```python
from build123d import *

# Parameters (mm, degrees)
F0_R     = 1.4
F1_DEPTH = 40
F2_W     = 3.4122867597
F2_H     = 22.5
F3_DEPTH = 25
F5_DEPTH = 2.75
F4_R     = 1.75
F4_R_2   = 19
F6_DEPTH = 25


with BuildPart() as f1:
    # F0 (on Top) → F1 (new body)
    with BuildSketch(Plane.XY):
        Polygon((-1.5877132403, -2.75), (1.5877132403, -2.75), (3.17543, 0), (1.5877132403, 2.75), (-3.3508529611, 5.5), (-46.7631397208, 5.5), (-46.7631397208, 2.75), (-4.7631397208, 2.75), (-3.1754264805, 0), align=None)
        Circle(F0_R, mode=Mode.SUBTRACT)
    extrude(amount=F1_DEPTH)

    # F2 (on face) → F3 (cut)
    with BuildSketch(Plane(origin=(0, 5.5, 0), x_dir=(-1, 0, 0), z_dir=(0, 1, 0))):
        Polygon((6.7631397208, 40.8263410057), (-4.1816732138, 40.8263410057), (-4.1816732138, 17.5), (3.3508529611, 17.5), (3.3508529611, 40), (6.7631397208, 40), align=None)
        with Locations((5.056996341, 28.75)):
            Rectangle(F2_W, F2_H)
    extrude(amount=-F3_DEPTH, mode=Mode.SUBTRACT)

    # F4 (on face) → F5 (join)
    with BuildSketch(Plane.XZ.offset(-2.75)):
        with BuildLine():
            Line((-46.7631397208, 9.692235936), (-46.7631397208, 30.307764064))
            ThreePointArc((-46.7631397208, 30.307764064), (-49.2631397208, 20), (-46.7631397208, 9.692235936))
        make_face()
        with BuildLine():
            ThreePointArc((-16.4553756568, 40), (-26.7631397208, 42.5), (-37.0709037849, 40))
            Line((-37.0709037849, 40), (-16.4553756568, 40))
        make_face()
    extrude(amount=-F5_DEPTH)

    # F4 (on face) → F6 (cut)
    with BuildSketch(Plane.XZ.offset(-2.75)):
        with BuildLine():
            Line((-6.7631397208, 40), (-9.7631397208, 40))
            ThreePointArc((-9.7631397208, 40), (-7.6418193773, 39.1213203436), (-6.7631397208, 37))
            Line((-6.7631397208, 37), (-6.7631397208, 40))
        make_face()
        with BuildLine():
            ThreePointArc((-46.7631397208, 37), (-45.8844600644, 39.1213203436), (-43.7631397208, 40))
            Line((-43.7631397208, 40), (-46.7631397208, 40))
            Line((-46.7631397208, 40), (-46.7631397208, 37))
        make_face()
        with Locations((-42.6730422975, 35.9099025767)):
            Circle(F4_R)
        with Locations((-42.6730422975, 4.0900974233)):
            Circle(F4_R)
        with Locations((-10.8532371441, 4.0900974233)):
            Circle(F4_R)
        with Locations((-10.8532371441, 35.9099025767)):
            Circle(F4_R)
        with Locations((-26.7631397208, 20)):
            Circle(F4_R_2)
    extrude(amount=-F6_DEPTH, mode=Mode.SUBTRACT)


solid = f1.part
```
Geometry: final body of the model. Coordinates: model frame, mm. A direction names the side the tool comes from. Round coordinates to 2 decimals unless told otherwise and drop trailing zeros. Order: outer loops, then holes, each group sorted by start corner. A loop starts at its lowest first (then second) coordinate and runs counter-clockwise, first axis right, second up. Notation, with made-up numbers: (77, 20) -> (135, 20) arc R17 ccw to (135, 26) -> close; hole circle Ø6 at (33.25, 88.5). An arc over 180 degrees is marked (long way). Use CSV: the item, a comma, the result in double quotes. Start each with the question number.
1) Section B-B (z = 13). Return the cut outline in (x, y), and give its area (3 significant figures).
2) Section C-C (x = 0). Return the cut outline in (y, z).
3) Draft query along Z for faces 4 (the face through (-9.184, 4.106, 36.436)), 5 (the face through (-0.847, 4.106, 8.628)), 6 (the face through (-46, 4, 39)), 7 (the face through (-44.42, 4.11, 4.17)). Return one class per face: +Z half, -Z half, draft (parallel to the pull), parting line (faces both ways), or undercut.
4) Section D-D (y = 4.75). Return the cut outline in (x, z), and give its area (3 significant figures).
5) Section A-A (z = 20). Return the cut outline in (x, y), and give its area (3 significant figures).
6) Material intervals for line 1 along X through (y, z) = (4, 4); line 2 along X through (y, z) = (-0.75, 9); line 3 along X through (y, z) = (4.75, 7), sorted ascending. Write a range as from..to.
7) First-contact query: pin 1 Ø2 at (x, z) = (-42.67, 35.91) entering from -Y; pin 2 Ø4 at (x, z) = (-10.85, 35.91) entering from -Y; pin 3 Ø1.4 at (x, y) = (-40.5, 4.5) entering from +Z; pin 4 Ø2 at (y, z) = (4.5, 32.5) entering from -X. Flat tips, straight axial feed; report the tip coordinate or a pass-through.
8) Set-up query: faces 1 (the face through (2.39, 1.36, 8.63)), 2 (the face through (-13, 4, 40)), 3 (the face through (-46.763, 4, 34)). Return all of +Z, -Z, +X, -X, +Y, -Y with unobstructed straight access to the full face (end or side cutting, diameter ignored); none if empty.
Returned:
1,outline,"(-48.15, 2.75) -> (-44.43, 2.75) -> (-44.43, 5.5) -> (-48.15, 5.5) -> close; (-9.1, 2.75) -> (-4.76, 2.75) -> (-1.59, -2.75) -> (1.59, -2.75) -> (3.18, 0) -> (1.59, 2.75) -> (-3.35, 5.5) -> (-9.1, 5.5) -> close; hole circle Ø2.8 at (0, 0)"
1,area,"57.2 mm²"
2,outline,"(-2.75, 0) -> (-1.4, 0) -> (-1.4, 17.5) -> (-2.75, 17.5) -> close; (1.4, 0) -> (3.63, 0) -> (3.63, 17.5) -> (1.4, 17.5) -> close"
3,face 4,"undercut"
3,face 5,"draft"
3,face 6,"+Z half"
3,face 7,"undercut"
4,outline,"(-46.76, 0) -> (-2, 0) -> (-2, 17.5) -> (-6.76, 17.5) -> (-6.76, 37) arc R3 ccw to (-9.76, 40) -> (-16.46, 40) arc R22.5 ccw to (-37.07, 40) -> (-43.76, 40) arc R3 ccw to (-46.76, 37) -> (-46.76, 30.31) arc R22.5 ccw to (-46.76, 9.69) -> close; hole circle Ø38 at (-26.76, 20); hole circle Ø3.5 at (-42.67, 4.09); hole circle Ø3.5 at (-42.67, 35.91); hole circle Ø3.5 at (-10.85, 4.09); hole circle Ø3.5 at (-10.85, 35.91)"
4,area,"576 mm²"
5,outline,"(-49.26, 2.75) -> (-45.76, 2.75) -> (-45.76, 5.5) -> (-49.26, 5.5) -> close; (-7.76, 2.75) -> (-6.76, 2.75) -> (-6.76, 5.5) -> (-7.76, 5.5) -> close"
5,area,"12.4 mm²"
6,line 1,"x = -46.76..-44.42, -40.93..-37.01, -16.52..-12.6, -9.11..-0.66"
6,line 2,"x = -2.74..-1.18, 1.18..2.74"
6,line 3,"x = -46.76..-40.62, -12.91..-2"
7,pin 1,"passes through"
7,pin 2,"stops at y = 2.75"
7,pin 3,"stops at z = 40"
7,pin 4,"stops at x = -46.76"
8,face 1,"+Z, -Z, +X, +Y"
8,face 2,"+Z, +X, +Y, -Y"
8,face 3,"+Z, -X, +Y, -Y"
